```python
from build123d import *

# Parameters (mm, degrees)
SKETCH1_R                                      = 19.05
BOSS_EXTRUDE1_DEPTH                            = 3.81
SKETCH2_R                                      = 12.6365
BOSS_EXTRUDE2_DEPTH                            = 1.27
CBORE_FOR_2_SOCKET_HEAD_CAP_SCREW1_D           = 2.4384
CBORE_FOR_2_SOCKET_HEAD_CAP_SCREW1_CBORE_D     = 4.7625
CBORE_FOR_2_SOCKET_HEAD_CAP_SCREW1_CBORE_DEPTH = 2.1844
CIRPATTERN1_COUNT                              = 5
F_1_8_0_1250_DOWEL_HOLE1_D                     = 3.175


with BuildPart() as part:
    # Sketch1 → Boss-Extrude1 (new body)
    with BuildSketch(Plane.XY):
        Circle(SKETCH1_R)
    extrude(amount=BOSS_EXTRUDE1_DEPTH)

    # Sketch2 → Boss-Extrude2 (add)
    with BuildSketch(Plane.XY.offset(3.81)):
        Circle(SKETCH2_R)
    extrude(amount=BOSS_EXTRUDE2_DEPTH)

    # CBORE for _2 Socket Head Cap Screw1 (through all)
    with Locations(Plane(origin=(0, 0, 0), x_dir=(-1, 0, 0), z_dir=(0, 0, -1))):
        with Locations((15.875, 0)):
            cbore_for_2_socket_head_cap_screw1 = CounterBoreHole(CBORE_FOR_2_SOCKET_HEAD_CAP_SCREW1_D / 2, CBORE_FOR_2_SOCKET_HEAD_CAP_SCREW1_CBORE_D / 2, CBORE_FOR_2_SOCKET_HEAD_CAP_SCREW1_CBORE_DEPTH)

    # CirPattern1: CBORE for _2 Socket Head Cap Screw1 ×5 about axis
    cirpattern1_axis = Axis((0, 0, 0), (0, 0, 1))
    for i in range(1, CIRPATTERN1_COUNT):
        add(cbore_for_2_socket_head_cap_screw1.rotate(cirpattern1_axis, i * 360 / CIRPATTERN1_COUNT), mode=Mode.SUBTRACT)

    # 1_8 _0.1250_ Dowel Hole1 (through all)
    with Locations(Plane(origin=(0, 0, 0), x_dir=(-1, 0, 0), z_dir=(0, 0, -1))):
        with Locations((0, 0)):
            Hole(F_1_8_0_1250_DOWEL_HOLE1_D / 2)


solid = part.part
```
Check sheet for the modelled part. Datum: model origin and axes. Units: mm. A direction names the side the tool comes from. Give positions to 0.01 mm unless a question says otherwise; leave off trailing zeros. Loops run counter-clockwise (first coordinate to the right, second up) from the corner with the lowest first, then second, coordinate; pieces in that order, holes last. Notation, with made-up numbers: M -32,38.25 L -20,38.25 A16 cw -20,47.25 Z; hole C 40.5,-37.75 d11. An arc over 180 degrees is marked long. Answer as CSV lines item,"result".
Item 1: Sectioned sample at C-C, the plane x = 13.5. Enter the section's corners in (y, z).
Reply:
outline,"M -13.44,0 L -11.62,0 L -11.62,2.18 L -10.36,2.18 L -10.36,3.81 L -13.44,3.81 Z; M -8.3,2.18 L -7.04,2.18 L -7.04,0 L 7.04,0 L 7.04,2.18 L 8.3,2.18 L 8.3,3.81 L -8.3,3.81 Z; M 10.36,2.18 L 11.62,2.18 L 11.62,0 L 13.44,0 L 13.44,3.81 L 10.36,3.81 Z"
Item 2: Depth check by flat-ended pin: pin 1 Ø3 at (x, y) = (-15.875, 0) entering from -Z; pin 2 Ø2 at (x, z) = (6, 3) entering from -Y; pin 3 Ø3 at (x, y) = (-4.91, -15.1) entering from +Z. Enter the tip coordinate at first touch or a pass-through.
Reply:
pin 1,"z = 2.18"
pin 2,"y = -18.38"
pin 3,"z = 3.81"
Item 3: Draft check along X on faces 4 (the face through (-6, -14, 2.184)), 5 (the face through (0, -4, 0)), 6 (the face through (-15.12, -11.59, 1.88)). Enter one of: pulls with the +X half, pulls with the -X half, needs draft (parallel to the pull), parting line crosses it, or undercut.
Reply:
face 4,"undercut"
face 5,"needs draft"
face 6,"parting line crosses it"
Item 4: Set-up check for faces 1 (the face through (-13, 0, 3.81)), 2 (the face through (13.86, 10.004, 3.009)), 3 (the face through (-17, -1, 2.184)): record each of +Z, -Z, +X, -X, +Y, -Y from which the full face is reachable in a straight line by a thin tool's end or side.
Reply:
face 1,"+Z"
face 2,"+Z, -Z"
face 3,"-Z"
Item 5: Sectioned sample at D-D, the plane z = 4.25. Enter the section's corners in (x, y) (1 decimal).
Reply:
outline,"C 0,0 d25.3; hole C 0,0 d3.2"
Item 6: Scan lines: L1, parallel to X at y = 0.5, z = 2.9; L2, parallel to Z at x = -12, y = -6; L3, parallel to X at y = -14, z = 2.55. Record each from-to range of solid material in increasing order.
Reply:
L1,"-19.04 to -16.99, -14.76 to -1.51, 1.51 to 19.04"
L2,"0 to 3.81"
L3,"-12.92 to -5.44, -4.38 to 12.92"
Item 7: Sectioned sample at A-A, the plane y = 0. Enter the section's corners in (x, z), then the cut area to 3 significant figures.
Reply:
outline,"M -19.05,0 L -18.26,0 L -18.26,2.18 L -17.09,2.18 L -17.09,3.81 L -19.05,3.81 Z; M -14.66,2.18 L -13.49,2.18 L -13.49,0 L -1.59,0 L -1.59,5.08 L -12.64,5.08 L -12.64,3.81 L -14.66,3.81 Z; M 1.59,0 L 19.05,0 L 19.05,3.81 L 12.64,3.81 L 12.64,5.08 L 1.59,5.08 Z"
area,"147 mm^2"
Item 8: Sectioned sample at B-B, the plane x = 0. Enter the section's corners in (y, z).
Reply:
outline,"M -19.05,0 L -1.59,0 L -1.59,5.08 L -12.64,5.08 L -12.64,3.81 L -19.05,3.81 Z; M 1.59,0 L 19.05,0 L 19.05,3.81 L 12.64,3.81 L 12.64,5.08 L 1.59,5.08 Z"
